Can you work these out from the drawing? Everything is in mm from the part's minimum corner. Coordinates: 2 decimals unless noted, no trailing zeros. Loops run counter-clockwise (first coordinate to the right, second up) from the corner with the lowest first, then second, coordinate; pieces in that order, holes last. Notation, with made-up numbers: (61.25, 62) - (77.25, 62) arc R24 cw to (77.25, 99) - close; hole circle Ø2 at (86, 32). An arc over 180 degrees is marked (long way). Use CSV: the item, a comma, the result in double quotes.
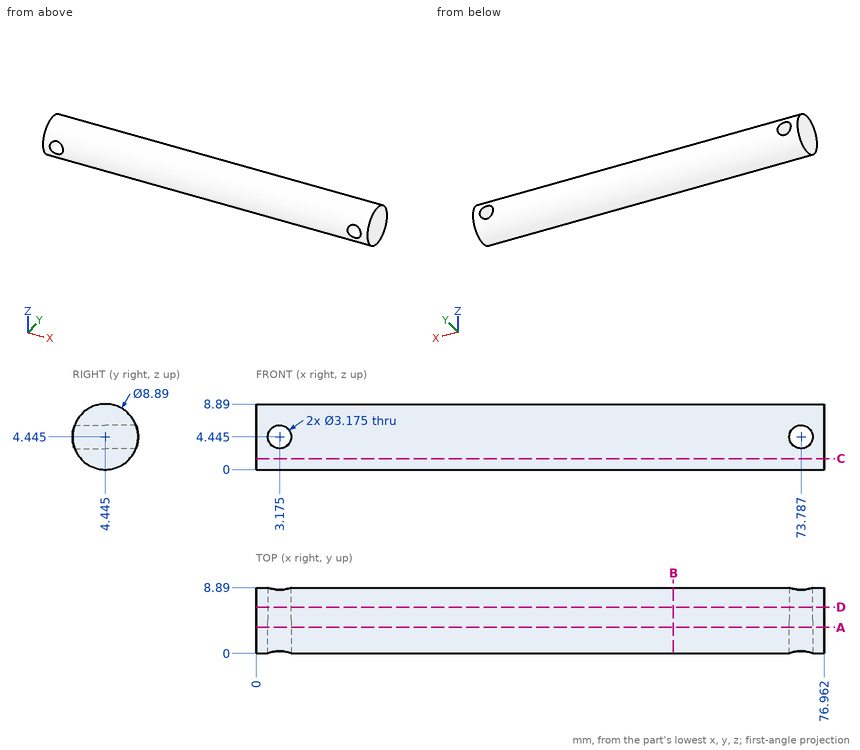
(1) Suppose I cut it at B-B (x = 56.5). Write out the boundary of the cut face in (y, z) (3 decimals), plus the area to 3 significant figures.
Computed:
outline,"circle Ø8.89 at (4.445, 4.445)"
area,"62.1 mm²"
(2) Suppose I cut it at C-C (z = 1.5). Write out the boundary of the cut face in (x, y).
Computed:
outline,"(0, 1.12) - (76.96, 1.12) - (76.96, 7.77) - (0, 7.77) - close"
(3) Will these pins go through, and if not, where does the flat tip stop? pin 1 (1.5 mm diameter, centred on x = 47, z = 7, fed in from -Y); pin 2 (5 mm diameter, centred on x = 16.5, z = 1.5, fed in from +Y).
Computed:
pin 1,"stops at y = 0.38"
pin 2,"stops at y = 8.87"
(4) Please list where these lines run through material, in increasing order: line 1 (X direction, y = 7.5, z = 3); line 2 (X direction, y = 7.25, z = 5.75); line 3 (Z direction, x = 31, y = 7.75).
Computed:
line 1,"x = 0 to 2.52, 3.83 to 73.13, 74.44 to 76.96"
line 2,"x = 0 to 2.27, 4.08 to 72.88, 74.69 to 76.96"
line 3,"z = 1.47 to 7.42"
(5) Suppose I cut it at A-A (y = 3.5). Write out the boundary of the cut face in (x, z) (1 decimal), plus the area to 3 significant figures.
Computed:
outline,"(0, 0.1) - (77, 0.1) - (77, 8.8) - (0, 8.8) - close; hole circle Ø3.2 at (3.2, 4.4); hole circle Ø3.2 at (73.8, 4.4)"
area,"653 mm²"
(6) Suppose I cut it at D-D (y = 6.25). Write out the boundary of the cut face in (x, z) (1 decimal).
Computed:
outline,"(0, 0.4) - (77, 0.4) - (77, 8.5) - (0, 8.5) - close; hole circle Ø3.2 at (3.2, 4.4); hole circle Ø3.2 at (73.8, 4.4)"
